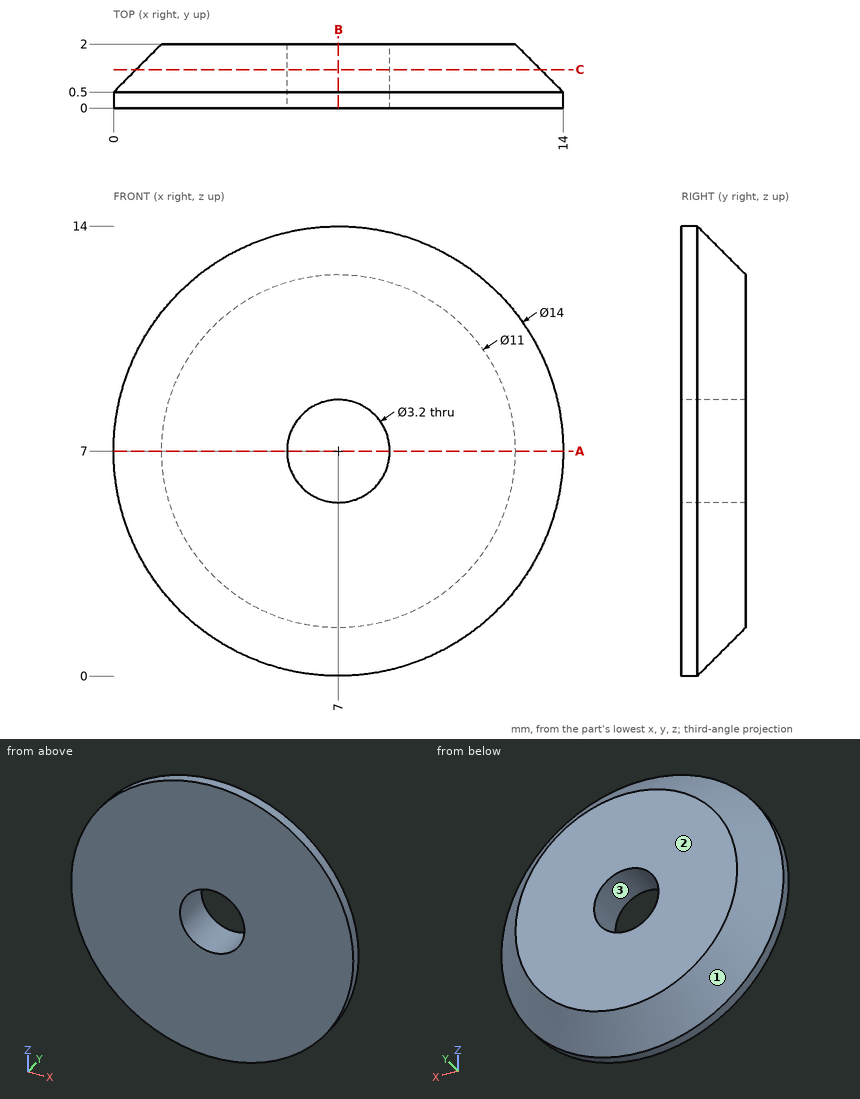
Design review of the part shown in the three views and the two pictorial views. Dimensions are in mm from the part's minimum x, y and z. Round coordinates to 2 decimals unless told otherwise and drop trailing zeros. Write each loop counter-clockwise with the first axis right and the second up, starting at its lowest first coordinate (ties: lowest second). Pieces come first, ordered by that corner, then holes. Notation, with made-up numbers: (47, 88.5) -> (63, 88.5) arc R14 cw to (63, 99.5) -> close; hole circle Ø7 at (8, 10.25). An arc over 180 degrees is marked (long way). Use one line per item in the form item = value.
1) Take a section at B-B, the plane x = 7. Write out the cut boundary in (y, z).
Found:
outline = (0, 0) -> (0.5, 0) -> (2, 1.5) -> (2, 5.4) -> (0, 5.4) -> close; (0, 8.6) -> (2, 8.6) -> (2, 12.5) -> (0.5, 14) -> (0, 14) -> close
2) Clearance check with flat-ended pins moving along their axes: pin 1 (1.5 mm diameter, centred on x = 8.5, z = 11.5, fed in from -Y); pin 2 (1 mm diameter, centred on x = 2, y = 0.5, fed in from +Z). State where each tip first meets the part, or that it passes through.
Found:
pin_1 = 0
pin_2 = 12.36
3) To check wall thickness, follow L1, parallel to Z at x = 7, y = 0.7; L2, parallel to Z at x = 7, y = 0.6; L3, parallel to Y at x = 3.5, z = 11.75. State the ranges of each line that lie inside material, in increasing order. Write a range as from..to.
Found:
L1 = 0.2..5.4, 8.6..13.8
L2 = 0.1..5.4, 8.6..13.9
L3 = 0..1.6
4) Take a section at C-C, the plane y = 1.2. Write out the cut boundary in (x, z).
Found:
outline = circle Ø12.6 at (7, 7); hole circle Ø3.2 at (7, 7)
5) Mouldability with a two-part tool opening along Z and no side actions: class the marked faces 1, 2 and 3 as +Z half, -Z half, draft (parallel to the pull), parting line (faces both ways), or undercut.
Found:
face_1 = parting line
face_2 = draft
face_3 = undercut
6) Take a section at A-A, the plane z = 7. Write out the cut boundary in (x, y), and give its area (4 significant figures).
Found:
outline = (0, 0) -> (5.4, 0) -> (5.4, 2) -> (1.5, 2) -> (0, 0.5) -> close; (8.6, 0) -> (14, 0) -> (14, 0.5) -> (12.5, 2) -> (8.6, 2) -> close
area = 19.35 mm2
